```python
from build123d import *

# Parameters (mm, degrees)
SKETCH4_W          = 958.607886296
SKETCH4_H          = 357.948466727
CUT_EXTRUDE2_DEPTH = 620
SKETCH5_W          = 348.415387901
SKETCH5_H          = 679.160017281
SKETCH5_W_2        = 379.676333146
SKETCH5_H_2        = 859.178335114
CUT_EXTRUDE3_DEPTH = 500


with BuildPart() as part:
    # Sketch1 → Revolve1 (revolve)
    with BuildSketch(Plane(origin=(0, 0, 0), x_dir=(1, 0, 0), z_dir=(0, 1, 0)), mode=Mode.PRIVATE) as revolve1_sk:
        with BuildLine():
            Line((-38.416122965, -102.435963202), (581.583877035, -102.435963202))
            add(Edge.make_bspline(
                [(581.583877035, -102.435963202), (693.455539681, -103.300064727), (691.583877035, -210.80239754), (691.583877035, -232.435963192)],
                knots=[0, 0, 0, 0, 1, 1, 1, 1], degree=3))
            Line((691.583877035, -232.435963192), (688.583877035, -232.435963192))
            add(Edge.make_bspline(
                [(581.572240946, -105.435963202), (582.424150652, -105.442600659), (584.137918536, -105.468851395), (587.484086921, -105.571526796), (591.571096113, -105.792916991), (596.307608869, -106.20262694), (602.409126826, -106.934758126), (609.639419087, -108.18665603), (617.705857071, -110.190510236), (625.186745256, -112.659295822), (634.414245375, -116.523312816), (644.612073728, -122.339029978), (654.913796392, -130.630357057), (663.469285855, -139.982021209), (670.450391217, -150.141502012), (676.016737994, -160.847618745), (680.323342136, -171.829037867), (683.525745861, -182.806951112), (685.782094183, -193.498408861), (687.253383878, -203.618874424), (687.961369137, -211.339785332), (688.299442483, -216.947462036), (688.459593049, -220.834002423), (688.547117141, -224.365875375), (688.582824389, -227.512914091), (688.58674237, -229.777140481), (688.584795317, -231.383827189), (688.583877035, -232.075985649), (688.583877035, -232.435963192)],
                knots=[3.4973e-05, 3.4973e-05, 3.4973e-05, 3.4973e-05, 0.0078472, 0.015659426, 0.03128388, 0.046908334, 0.062532787, 0.093781694, 0.125030601, 0.156279508, 0.187528415, 0.25002623, 0.312524044, 0.375021858, 0.437519672, 0.500017486, 0.562515301, 0.625013115, 0.687510929, 0.750008743, 0.812506557, 0.843755465, 0.875004372, 0.906253279, 0.937502186, 0.968751093, 0.984375546, 1, 1, 1, 1], degree=3))
            Line((581.572240946, -105.435963202), (-38.416122951, -105.435969803))
            add(Edge.make_bspline(
                [(-145.416150087, -297.448719694), (-145.415786094, -297.363118797), (-145.414261278, -297.209117302), (-145.406482156, -296.763589127), (-145.387577621, -296.059017238), (-145.348080967, -294.963719442), (-145.270536885, -293.196191663), (-145.12221169, -290.430217628), (-144.846888777, -286.292241124), (-144.459106758, -281.402026013), (-143.771963774, -273.967299792), (-142.556325425, -263.124157442), (-140.406308296, -248.159348272), (-137.445210779, -231.767940973), (-133.55430361, -214.477141353), (-128.616651259, -196.81526366), (-122.518262583, -179.311948455), (-115.149922932, -162.497881736), (-106.409989847, -146.903194531), (-96.207058742, -133.05233616), (-86.417989624, -123.386032183), (-77.769632288, -117.014146282), (-70.859172034, -112.970513688), (-63.504748075, -109.716446776), (-56.985343251, -107.708604585), (-51.52041341, -106.554160283), (-47.294097057, -105.922162765), (-43.659473987, -105.597170774), (-40.689467236, -105.462466746), (-39.171234927, -105.437583269), (-38.416122951, -105.435969803)],
                knots=[2.115e-05, 2.115e-05, 2.115e-05, 2.115e-05, 0.007833485, 0.015645819, 0.031270489, 0.046895159, 0.062519828, 0.093769167, 0.125018506, 0.156267845, 0.187517184, 0.250015862, 0.312514541, 0.375013219, 0.437511897, 0.500010575, 0.562509253, 0.625007931, 0.687506609, 0.750005287, 0.812503966, 0.843753305, 0.875002644, 0.906251983, 0.937501322, 0.953125991, 0.968750661, 0.98437533, 0.992187665, 1, 1, 1, 1], degree=3))
            Line((-145.416150087, -297.448719694), (-148.416122965, -297.435963202))
            add(Edge.make_bspline(
                [(-38.416122965, -102.435963202), (-139.444928363, -102.64405425), (-148.369931417, -286.57299354), (-148.416122965, -297.435963202)],
                knots=[0, 0, 0, 0, 1, 1, 1, 1], degree=3))
        make_face()
    revolve(revolve1_sk.sketch.rotate(Axis((-396.592099756, 0, 312.435963202), (1, 0, 0)), 180), axis=Axis((-396.592099756, 0, 312.435963202), (1, 0, 0)))

    # Sketch4 → Cut-Extrude2 (cut)
    with BuildSketch(Plane(origin=(-38.416122965, 0, 0), x_dir=(0, 0, -1), z_dir=(1, 0, 0))):
        with Locations((-258.191988159, 178.974233364)):
            Rectangle(SKETCH4_W, SKETCH4_H)
    extrude(amount=CUT_EXTRUDE2_DEPTH, mode=Mode.SUBTRACT)

    # Sketch5 → Cut-Extrude3 (cut, symmetric)
    with BuildSketch(Plane(origin=(0, 0, 0), x_dir=(1, 0, 0), z_dir=(0, 1, 0))):
        with Locations((-212.623816916, -235.263662883)):
            Rectangle(SKETCH5_W, SKETCH5_H)
        with Locations((771.422043608, -306.861857476)):
            Rectangle(SKETCH5_W_2, SKETCH5_H_2)
    extrude(amount=CUT_EXTRUDE3_DEPTH, both=True, mode=Mode.SUBTRACT)


solid = part.part
```
Model file for the job. Use its own axes, mm. Coordinates: 2 decimals unless noted, no trailing zeros. Write each loop counter-clockwise with the first axis right and the second up, starting at its lowest first coordinate (ties: lowest second). Pieces come first, ordered by that corner, then holes. Notation, with made-up numbers: (18.25, 14) - (69.25, 14) arc R25 cw to (69.25, 31) - close; hole circle Ø3 at (78, -20). An arc over 180 degrees is marked (long way). Use a Markdown table: item, result. Add a question column.
Item 1: Drop flat-ended pins along their axis: pin 1 (5 mm diameter, centred on x = 79.5, z = 204.5, fed in from +Y); pin 2 (1 mm diameter, centred on x = 363.5, y = -82.5, fed in from +Z); pin 3 (4 mm diameter, centred on x = 251, y = -152.5, fed in from -Z). Give the stop position or say it passes through.
Item 2: Drill centre lines: line 1 along Z through (x, y) = (82.5, -146); line 2 along Z through (x, y) = (515, -155.5); line 3 along Y through (x, z) = (520, 433). Where is each one in solid material? Low to high.
Item 3: Two-plate mould, pull along Z, no slides. Class faces 1 (the face through (275.92, -209.95, 317.05)), 2 (the face through (267.24, -206.95, 316.99)), 3 (the face through (-38.416, -207, 329)): pulls with the +Z half, pulls with the -Z half, needs draft (parallel to the pull), parting line crosses it, or undercut.
Item 4: Band-saw the part on A-A, the plane x = 414.5. Write the cut outline in (y, z), and give its area (3 significant figures).
A:
| question | item | result |
|---|---|---|
| 1 | pin 1 | stops at y = -175.08 |
| 1 | pin 2 | stops at z = 505.76 |
| 1 | pin 3 | stops at z = 165.98 |
| 2 | line 1 | z = 161.49 to 165.69, 459.18 to 463.38 |
| 2 | line 2 | z = 171.3 to 175.8, 449.07 to 453.57 |
| 2 | line 3 | y = -171.94 to -168.27 |
| 3 | face 1 | parting line crosses it |
| 3 | face 2 | undercut |
| 3 | face 3 | needs draft |
| 4 | outline | (0, 102.44) - (0, 105.44) arc R207 cw to (0, 519.44) - (0, 522.44) arc R210 ccw to start |
| 4 | area | 1,970 mm² |
